Design review of the part built by this model. Coordinates are the model's own, in mm. A direction names the side the tool comes from. Give positions to 0.01 mm unless a question says otherwise; leave off trailing zeros. Write each loop counter-clockwise with the first axis right and the second up, starting at its lowest first coordinate (ties: lowest second). Pieces come first, ordered by that corner, then holes. Notation, with made-up numbers: (16.5, 78.25) -> (63.5, 78.25) arc R21 ccw to (63.5, 83.25) -> close; hole circle Ø11 at (76.25, 15.25). An arc over 180 degrees is marked (long way). Use CSV: the item, a comma, the result in double quotes.
```python
from build123d import *

# Parameters (mm, degrees)
BOSS_EXTRUDE1_DEPTH = 6.35


with BuildPart() as part:
    # Model → Boss-Extrude1 (new body)
    with BuildSketch(Plane.XY):
        with BuildLine():
            Line((32021.317821572, 25274.323174378), (31898.42286363, 25349.042544488))
            ThreePointArc((31898.42286363, 25349.042544488), (31894.462469578, 25357.265056675), (31900.359077013, 25364.231005892))
            ThreePointArc((31900.359077013, 25364.231005892), (31948.042704711, 25400.357680634), (31981.621767845, 25449.868401671))
            ThreePointArc((31981.621767845, 25449.868401671), (32006.341646593, 25570.177684815), (32000.625291763, 25692.867208832))
            ThreePointArc((32000.625291763, 25692.867208832), (31975.507241516, 25856.663875176), (31968.102557494, 26022.209744977))
            ThreePointArc((31968.102557494, 26022.209744977), (31962.641360506, 26062.007077803), (31944.412049452, 26097.802951743))
            ThreePointArc((31944.412049452, 26097.802951743), (31943.68670031, 26101.762571322), (31944.890892918, 26105.603748061))
            ThreePointArc((31944.890892918, 26105.603748061), (31947.746914305, 26108.440623176), (31951.596103907, 26109.618951649))
            ThreePointArc((31951.596103907, 26109.618951649), (31991.765349883, 26109.908866112), (32029.610966233, 26123.375925767))
            ThreePointArc((32029.610966233, 26123.375925767), (32179.991169477, 26192.989565418), (32336.970470479, 26246.072174717))
            ThreePointArc((32336.970470479, 26246.072174717), (32429.228020558, 26286.060888433), (32511.480316916, 26343.897836094))
            ThreePointArc((32511.480316916, 26343.897836094), (32528.070496221, 26358.968782526), (32543.960172601, 26374.776554672))
            ThreePointArc((32543.960172601, 26374.776554672), (32572.462265233, 26427.374042198), (32582.590731747, 26486.334021375))
            ThreePointArc((32582.590731747, 26486.334021375), (32584.378351728, 26493.233188238), (32590.829278865, 26496.262978274))
            Line((32590.829278865, 26496.262978274), (32660.015563019, 26496.262978274))
            Line((32660.015563019, 26496.262978274), (32729.201847174, 26496.262978274))
            ThreePointArc((32729.201847174, 26496.262978274), (32735.652774311, 26493.233188238), (32737.440394292, 26486.334021375))
            ThreePointArc((32737.440394292, 26486.334021375), (32747.568860806, 26427.374042198), (32776.070953438, 26374.776554672))
            ThreePointArc((32776.070953438, 26374.776554672), (32791.960629818, 26358.968782526), (32808.550809123, 26343.897836094))
            ThreePointArc((32808.550809123, 26343.897836094), (32890.803105481, 26286.060888433), (32983.06065556, 26246.072174717))
            ThreePointArc((32983.06065556, 26246.072174717), (33140.039956563, 26192.989565418), (33290.420159808, 26123.375925766))
            ThreePointArc((33290.420159808, 26123.375925766), (33328.265776157, 26109.908866112), (33368.435022132, 26109.618951649))
            ThreePointArc((33368.435022132, 26109.618951649), (33372.284211734, 26108.440623176), (33375.140233121, 26105.603748061))
            ThreePointArc((33375.140233121, 26105.603748061), (33376.344425729, 26101.762571322), (33375.619076587, 26097.802951743))
            ThreePointArc((33375.619076587, 26097.802951743), (33357.389765533, 26062.007077803), (33351.928568545, 26022.209744977))
            ThreePointArc((33351.928568545, 26022.209744977), (33344.523884523, 25856.663875176), (33319.405834276, 25692.867208832))
            ThreePointArc((33319.405834276, 25692.867208832), (33313.689479446, 25570.177684815), (33338.409358194, 25449.868401671))
            ThreePointArc((33338.409358194, 25449.868401671), (33371.988421328, 25400.357680634), (33419.672049026, 25364.231005892))
            ThreePointArc((33419.672049026, 25364.231005892), (33425.568656461, 25357.265056675), (33421.608262409, 25349.042544488))
            Line((33421.608262409, 25349.042544488), (33298.713304467, 25274.323174378))
            Line((33298.713304467, 25274.323174378), (33175.818346525, 25199.603804268))
            ThreePointArc((33175.818346525, 25199.603804268), (33166.695707373, 25199.871913635), (33163.225042079, 25208.312820585))
            ThreePointArc((33163.225042079, 25208.312820585), (33153.096575565, 25267.272799762), (33124.594482933, 25319.870287288))
            ThreePointArc((33124.594482933, 25319.870287288), (33108.704806552, 25335.678059434), (33092.114627248, 25350.749005866))
            ThreePointArc((33092.114627248, 25350.749005866), (33009.862330892, 25408.585953526), (32917.604780817, 25448.574667241))
            ThreePointArc((32917.604780817, 25448.574667241), (32820.801117373, 25479.077054216), (32726.212567172, 25515.878562856))
            ThreePointArc((32726.212567172, 25515.878562856), (32693.800758918, 25525.993933375), (32660.015563019, 25529.371295238))
            ThreePointArc((32660.015563019, 25529.371295238), (32626.230367121, 25525.993933375), (32593.818558867, 25515.878562856))
            ThreePointArc((32593.818558867, 25515.878562856), (32499.230008667, 25479.077054216), (32402.426345225, 25448.574667242))
            ThreePointArc((32402.426345225, 25448.574667242), (32310.168795148, 25408.585953526), (32227.916498791, 25350.749005866))
            ThreePointArc((32227.916498791, 25350.749005866), (32211.326319487, 25335.678059434), (32195.436643106, 25319.870287288))
            ThreePointArc((32195.436643106, 25319.870287288), (32166.934550474, 25267.272799762), (32156.80608396, 25208.312820585))
            ThreePointArc((32156.80608396, 25208.312820585), (32153.335418666, 25199.871913635), (32144.212779514, 25199.603804268))
            Line((32144.212779514, 25199.603804268), (32021.317821572, 25274.323174378))
        make_face()
        with BuildLine():
            Line((32161.945371032, 25505.705998708), (32162.020964729, 25505.660038211))
            ThreePointArc((32162.020964729, 25505.660038211), (32176.714225147, 25498.923547863), (32192.565234673, 25495.758472672))
            ThreePointArc((32192.565234673, 25495.758472672), (32206.728801248, 25496.05984726), (32220.537857569, 25499.223296059))
            ThreePointArc((32220.537857569, 25499.223296059), (32355.626894288, 25538.977287334), (32487.434068472, 25588.538325436))
            ThreePointArc((32487.434068472, 25588.538325436), (32565.292000239, 25647.320716044), (32636.968512547, 25713.500052457))
            ThreePointArc((32636.968512547, 25713.500052457), (32647.52230753, 25720.62082965), (32660.01556302, 25723.071671069))
            ThreePointArc((32660.01556302, 25723.071671069), (32672.508818509, 25720.62082965), (32683.062613492, 25713.500052457))
            ThreePointArc((32683.062613492, 25713.500052457), (32754.7391258, 25647.320716043), (32832.597057568, 25588.538325434))
            ThreePointArc((32832.597057568, 25588.538325434), (32964.404231752, 25538.977287333), (33099.49326847, 25499.223296059))
            ThreePointArc((33099.49326847, 25499.223296059), (33113.302324791, 25496.059847259), (33127.465891366, 25495.758472671))
            ThreePointArc((33127.465891366, 25495.758472671), (33143.316900969, 25498.923547887), (33158.010161449, 25505.660038295))
            Line((33158.010161449, 25505.660038295), (33158.085755006, 25505.705998708))
            ThreePointArc((33158.085755006, 25505.705998708), (33179.843665848, 25526.578681224), (33190.730981851, 25554.695258361))
            ThreePointArc((33190.730981851, 25554.695258361), (33217.9002723, 25694.796891925), (33242.519614962, 25835.369030123))
            ThreePointArc((33242.519614962, 25835.369030123), (33238.20758577, 25922.098711206), (33205.875935233, 26002.692107648))
            ThreePointArc((33205.875935233, 26002.692107648), (33149.204409657, 26068.487011442), (33074.189865311, 26112.230003031))
            ThreePointArc((33074.189865311, 26112.230003031), (32897.241000802, 26167.38397641), (32719.040004698, 26218.347359521))
            ThreePointArc((32719.040004698, 26218.347359521), (32689.79224157, 26224.274724699), (32660.015563019, 26226.253289931))
            ThreePointArc((32660.015563019, 26226.253289931), (32630.238884468, 26224.274724699), (32600.991121341, 26218.347359521))
            ThreePointArc((32600.991121341, 26218.347359521), (32422.790125237, 26167.38397641), (32245.841260727, 26112.230003031))
            ThreePointArc((32245.841260727, 26112.230003031), (32170.826716382, 26068.487011443), (32114.155190805, 26002.692107648))
            ThreePointArc((32114.155190805, 26002.692107648), (32081.823540268, 25922.098711206), (32077.511511077, 25835.369030123))
            ThreePointArc((32077.511511077, 25835.369030123), (32102.130853739, 25694.796891925), (32129.300144187, 25554.695258362))
            ThreePointArc((32129.300144187, 25554.695258362), (32140.18746019, 25526.578681225), (32161.945371032, 25505.705998708))
        make_face(mode=Mode.SUBTRACT)
    extrude(amount=BOSS_EXTRUDE1_DEPTH)


solid = part.part
```
(1) For line 1 along X through (y, z) = (25636.5, 5); line 2 along X through (y, z) = (25676.5, 2.5); line 3 along Y through (x, z) = (32832.5, 4.5), list the stretches that pass through material, from the lowest coordinate up. Write a range as [from, to].
Established:
line 1,"x = [32007.06, 32113.12], [32552.11, 32767.92], [33206.92, 33312.97]"
line 2,"x = [32003.17, 32105.53], [32598.66, 32721.37], [33214.5, 33316.86]"
line 3,"y = [25475.02, 25588.6], [26186.43, 26324.39]"
(2) Mouldability with a two-part tool opening along X and no side actions: class faces 4 (the face through (32177.84, 26192.13, 3.13)), 5 (the face through (32899.73, 26166.64, 3.13)), 6 (the face through (33371.41, 25400.97, 3.13)) as +X half, -X half, draft (parallel to the pull), parting line (faces both ways), or undercut.
Established:
face 4,"-X half"
face 5,"undercut"
face 6,"+X half"
(3) Take a section at B-B (x = 32272.5). Write out the cut boundary in (y, z).
Established:
outline,"(25385.19, 0) -> (25513.24, 0) -> (25513.24, 6.35) -> (25385.19, 6.35) -> close; (26120.83, 0) -> (26226.54, 0) -> (26226.54, 6.35) -> (26120.83, 6.35) -> close"
(4) Clearance check with flat-ended pins moving along their axes: pin 1 (2 mm diameter, centred on y = 26323.5, z = 3.5, fed in from +X); pin 2 (3 mm diameter, centred on y = 25620, z = 4, fed in from -X). State where each tip first meets the part, or that it passes through.
Established:
pin 1,"stops at x = 32834.99"
pin 2,"stops at x = 32007.68"
(5) Tool access review of faces 1 (the face through (32101.77, 25696.76, 3.13)), 2 (the face through (33344.75, 25858.97, 3.13)), 3 (the face through (33153.37, 25266.48, 3.13)): name each direction out of +Z, -Z, +X, -X, +Y, -Y from which nothing blocks a thin tool from reaching the whole face with its end or side.
Established:
face 1,"+Z, -Z"
face 2,"+Z, -Z, +X"
face 3,"+Z, -Z, -Y"
(6) Take a section at A-A (y = 25793.5). Write out the cut boundary in (x, z), then the cut area to 3 significant figures.
Established:
outline,"(31983.06, 0) -> (32084.57, 0) -> (32084.57, 6.35) -> (31983.06, 6.35) -> close; (33235.46, 0) -> (33336.97, 0) -> (33336.97, 6.35) -> (33235.46, 6.35) -> close"
area,"1,290 mm2"
(7) Take a section at C-C (y = 26409.5). Write out the cut boundary in (x, z), then the cut area to 3 significant figures.
Established:
outline,"(32565.2, 0) -> (32754.83, 0) -> (32754.83, 6.35) -> (32565.2, 6.35) -> close"
area,"1,200 mm2"
